```python
from build123d import *

# Parameters (mm, degrees)
F1_DEPTH = 3
F2_R     = 1.5
F2_W     = 15
F2_H     = 0.5
F3_DEPTH = 35
F4_DEPTH = 25
F5_DEPTH = 35
F6_DEPTH = 27.5


with BuildPart() as f1:
    # F0 (on Top) → F1 (new body)
    with BuildSketch(Plane.XY):
        with BuildLine():
            Line((-17.5, 0), (-17.5, -7.5))
            Line((-17.5, -7.5), (17.5, -7.5))
            Line((17.5, -7.5), (17.5, 0))
            Line((17.5, 0), (10.35, 0))
            ThreePointArc((10.35, 0), (8.75, -1.6), (7.15, 0))
            Line((7.15, 0), (0, 0))
            Line((0, 0), (-7.15, 0))
            ThreePointArc((-7.15, 0), (-8.75, -1.6), (-10.35, 0))
            Line((-10.35, 0), (-17.5, 0))
        make_face()
        with BuildLine():
            Line((-17.5, 7.5), (-17.5, 0))
            Line((-17.5, 0), (-10.35, 0))
            ThreePointArc((-10.35, 0), (-8.75, 1.6), (-7.15, 0))
            Line((-7.15, 0), (0, 0))
            Line((0, 0), (7.15, 0))
            ThreePointArc((7.15, 0), (8.75, 1.6), (10.35, 0))
            Line((10.35, 0), (17.5, 0))
            Line((17.5, 0), (17.5, 7.5))
            Line((17.5, 7.5), (-17.5, 7.5))
        make_face()
    extrude(amount=F1_DEPTH)

    # F2 (on face) → F3 (join)
    with BuildSketch(Plane.YZ.offset(17.5)):
        with BuildLine():
            ThreePointArc((-11, -0.5), (-8.5251262658, 0.5251262658), (-7.5, 3))
            ThreePointArc((-7.5, 3), (-13.4748737342, 5.4748737342), (-11, -0.5))
        make_face()
        with Locations((-11, 3)):
            Circle(F2_R, mode=Mode.SUBTRACT)
        with BuildLine():
            Line((-7.5, 0), (-7.5, 3))
            ThreePointArc((-7.5, 3), (-8.5251262658, 0.5251262658), (-11, -0.5))
            Line((-11, -0.5), (-7.5, -0.5))
            Line((-7.5, -0.5), (-7.5, 0))
        make_face()
        with Locations((0, -0.25)):
            Rectangle(F2_W, F2_H)
    extrude(amount=-F3_DEPTH)

    # F4 (cut): faces of the model
    f4_faces = [f1.faces().sort_by_distance(p)[0] for p in [
        (-8.75, 0, 0),
        (8.75, 0, 0),
    ]]
    extrude(f4_faces, amount=-F4_DEPTH, mode=Mode.SUBTRACT)

    # F2 (on face) → F5 (cut)
    with BuildSketch(Plane.YZ.offset(17.5)):
        with BuildLine():
            ThreePointArc((-11, -0.5), (-8.5251262658, 0.5251262658), (-7.5, 3))
            ThreePointArc((-7.5, 3), (-13.4748737342, 5.4748737342), (-11, -0.5))
        make_face()
        with Locations((-11, 3)):
            Circle(F2_R, mode=Mode.SUBTRACT)
        with BuildLine():
            Line((-7.5, 0), (-7.5, 3))
            ThreePointArc((-7.5, 3), (-8.5251262658, 0.5251262658), (-11, -0.5))
            Line((-11, -0.5), (-7.5, -0.5))
            Line((-7.5, -0.5), (-7.5, 0))
        make_face()
    extrude(amount=-F5_DEPTH, mode=Mode.SUBTRACT)

    # F2 (on face) → F6 (join)
    with BuildSketch(Plane.YZ.offset(17.5)):
        with BuildLine():
            ThreePointArc((-11, -0.5), (-8.5251262658, 0.5251262658), (-7.5, 3))
            ThreePointArc((-7.5, 3), (-13.4748737342, 5.4748737342), (-11, -0.5))
        make_face()
        with Locations((-11, 3)):
            Circle(F2_R, mode=Mode.SUBTRACT)
        with BuildLine():
            Line((-7.5, 0), (-7.5, 3))
            ThreePointArc((-7.5, 3), (-8.5251262658, 0.5251262658), (-11, -0.5))
            Line((-11, -0.5), (-7.5, -0.5))
            Line((-7.5, -0.5), (-7.5, 0))
        make_face()
    extrude(amount=-F6_DEPTH)


solid = f1.part
```
Can you work these out from the model? Positions are in its coordinate system, mm. A direction names the side the tool comes from. Round coordinates to 2 decimals unless told otherwise and drop trailing zeros. Loops run counter-clockwise (first coordinate to the right, second up) from the corner with the lowest first, then second, coordinate; pieces in that order, holes last. Notation, with made-up numbers: M 40,-35.75 L 48,-35.75 A13 cw 48,-17.75 Z; hole C -3.5,-19 d7. An arc over 180 degrees is marked long. Answer in a Markdown table with one row per item.
1. If we section it at C-C, the plane z = 3.5: Please give me the cut outline in (x, y).
Established:
| item | result |
|---|---|
| outline | M -10,-14.46 L 17.5,-14.46 L 17.5,-12.41 L -10,-12.41 Z; M -10,-9.59 L 17.5,-9.59 L 17.5,-7.54 L -10,-7.54 Z |
2. On a 3-axis mill with a long thin cutter (end or side, diameter ignored), from which of +Z, -Z, +X, -X, +Y, -Y can I reach the whole of each face in a straight line? I mean faces 4 (the face through (-17.5, 0, 1)), 5 (the face through (-10, -9, 3)), 6 (the face through (0, 0, 3)). Say none if no direction works.
Established:
| item | result |
|---|---|
| face 4 | +Z, -Z, -X, +Y, -Y |
| face 5 | +Z, -Z, -X, -Y |
| face 6 | +Z, +X, -X, +Y |
3. If we section it at D-D, the plane x = -0.5: Please give me the cut outline in (y, z), plus the area to 3 significant figures.
Established:
| item | result |
|---|---|
| outline | M -11,-0.5 L 7.5,-0.5 L 7.5,3 L -7.5,3 A3.5 ccw long Z; hole C -11,3 d3 |
| area | 86.5 mm² |
4. Thinking about a two-plate mould opening in Y: for faces 1 (the face through (10.35, 0.07, 1.23)), 2 (the face through (17.5, -6, 2)), 3 (the face through (-14, -7.5, 1)), which applies, pulls with the +Y half, pulls with the -Y half, needs draft (parallel to the pull), parting line crosses it, or undercut?
Established:
| item | result |
|---|---|
| face 1 | undercut |
| face 2 | needs draft |
| face 3 | pulls with the -Y half |
5. Please list where these lines run through material, in increasing order: line 1 (X direction, y = 0, z = 1.15); line 2 (Y direction, x = -8.75, z = 2); line 3 (Z direction, x = 5.75, y = -11). Write a range as from..to.
Established:
| item | result |
|---|---|
| line 1 | -17.5..-10.35, -7.15..7.15, 10.35..17.5 |
| line 2 | -14.35..-12.12, -9.88..-1.6, 1.6..7.5 |
| line 3 | -0.5..1.5, 4.5..6.5 |
6. I'm going to push flat-ended pins straight in: pin 1 Ø5 at (x, y) = (-8.75, 0) entering from +Z; pin 2 Ø3 at (x, z) = (-13, 1) entering from -Y; pin 3 Ø3.5 at (y, z) = (-9.5, 4.5) entering from -X. Where does each tip first touch, or does it pass through?
Established:
| item | result |
|---|---|
| pin 1 | z = 3 |
| pin 2 | y = -7.5 |
| pin 3 | x = -10 |
7. If we section it at B-B, the plane y = 0: Please give me the cut outline in (x, z), plus the area to 3 significant figures.
Established:
| item | result |
|---|---|
| outline | M -17.5,-0.5 L -10.35,-0.5 L -10.35,3 L -17.5,3 Z; M -7.15,-0.5 L 7.15,-0.5 L 7.15,3 L -7.15,3 Z; M 10.35,-0.5 L 17.5,-0.5 L 17.5,3 L 10.35,3 Z |
| area | 100 mm² |
8. If we section it at A-A, the plane x = -8.75: Please give me the cut outline in (y, z).
Established:
| item | result |
|---|---|
| outline | M -11,-0.5 L -1.6,-0.5 L -1.6,3 L -7.5,3 A3.5 ccw long Z; M 1.6,-0.5 L 7.5,-0.5 L 7.5,3 L 1.6,3 Z; hole C -11,3 d3 |
